```python
from build123d import *

# Parameters (mm, degrees)
F0_W     = 200
F0_H     = 200
F2_DEPTH = 0.5
F1_R     = 10
F3_DEPTH = 10


# Not quite as in the source:
# - a fillet or chamfer that OpenCascade refuses, or shapes differently, is made with other operations: its cross-section is extruded or revolved along the edge and cut away or added


with BuildPart() as f2:
    # F0 (on Top) → F2 (new body)
    with BuildSketch(Plane.XY):
        Rectangle(F0_W, F0_H)
    extrude(amount=F2_DEPTH)

    # F1 (on face) → F3 (join)
    with BuildSketch(Plane.XY):
        with Locations((-55, -20)):
            Circle(F1_R)
        with Locations((-15, 20)):
            Circle(F1_R)
        with Locations((25, -60)):
            Circle(F1_R)
        with Locations((25, 20)):
            Circle(F1_R)
        with Locations((65, -20)):
            Circle(F1_R)
        with Locations((65, 20)):
            Circle(F1_R)
    extrude(amount=F3_DEPTH)

    # F4: fillet of radius 10 on 6 edges, made by hand

    # F4_s1 → F4_t2 (revolve, cut)
    with BuildSketch(Plane.XZ.offset(20)):
        with BuildLine():
            ThreePointArc((-45, 0.5), (-48.0954678017, 7.2456883731), (-54.9874921777, 10))
            Line((-54.9874921777, 10), (-45, 10))
            Line((-45, 10), (-45, 0.5))
        make_face()
    revolve(axis=Axis((-55, -20, 10), (0, 0, 1)), mode=Mode.SUBTRACT)

    # F4_s3 → F4_t4 (revolve, cut)
    with BuildSketch(Plane.XZ.offset(-20)):
        with BuildLine():
            ThreePointArc((-5, 0.5), (-8.0954678017, 7.2456883731), (-14.9874921777, 10))
            Line((-14.9874921777, 10), (-5, 10))
            Line((-5, 10), (-5, 0.5))
        make_face()
    revolve(axis=Axis((-15, 20, 10), (0, 0, 1)), mode=Mode.SUBTRACT)

    # F4_s5 → F4_t6 (revolve, cut)
    with BuildSketch(Plane.XZ.offset(-20)):
        with BuildLine():
            ThreePointArc((35, 0.5), (31.9045321983, 7.2456883731), (25.0125078223, 10))
            Line((25.0125078223, 10), (35, 10))
            Line((35, 10), (35, 0.5))
        make_face()
    revolve(axis=Axis((25, 20, 10), (0, 0, 1)), mode=Mode.SUBTRACT)

    # F4_s7 → F4_t8 (revolve, cut)
    with BuildSketch(Plane.XZ.offset(-20)):
        with BuildLine():
            ThreePointArc((75, 0.5), (71.9045321983, 7.2456883731), (65.0125078223, 10))
            Line((65.0125078223, 10), (75, 10))
            Line((75, 10), (75, 0.5))
        make_face()
    revolve(axis=Axis((65, 20, 10), (0, 0, 1)), mode=Mode.SUBTRACT)

    # F4_s9 → F4_t10 (revolve, cut)
    with BuildSketch(Plane.XZ.offset(20)):
        with BuildLine():
            ThreePointArc((75, 0.5), (71.9045321983, 7.2456883731), (65.0125078223, 10))
            Line((65.0125078223, 10), (75, 10))
            Line((75, 10), (75, 0.5))
        make_face()
    revolve(axis=Axis((65, -20, 10), (0, 0, 1)), mode=Mode.SUBTRACT)

    # F4_s11 → F4_t12 (revolve, cut)
    with BuildSketch(Plane.XZ.offset(60)):
        with BuildLine():
            ThreePointArc((35, 0.5), (31.9045321983, 7.2456883731), (25.0125078223, 10))
            Line((25.0125078223, 10), (35, 10))
            Line((35, 10), (35, 0.5))
        make_face()
    revolve(axis=Axis((25, -60, 10), (0, 0, 1)), mode=Mode.SUBTRACT)


solid = f2.part
```
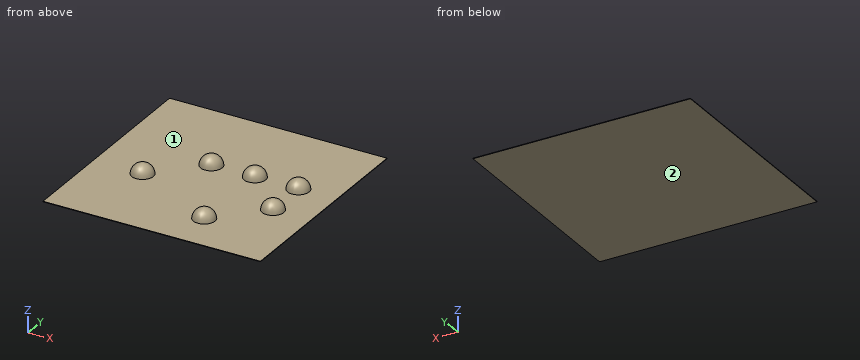
Here's how the part is built. I have some questions about the finished solid (model axes, mm). Face numbers are marked on the shaded views. A direction names the side the tool comes from. Round coordinates to 2 decimals unless told otherwise and drop trailing zeros. Loops run counter-clockwise (first coordinate to the right, second up) from the corner with the lowest first, then second, coordinate; pieces in that order, holes last.
1. Suppose I cut it at B-B, the plane z = 6.5. Give the number of separate pieces and of enclosed holes in the cut face, and give its area (3 significant figures).
Answers:
separate pieces: 6
enclosed holes: 0
area: 1,090 mm2
2. For the marked faces 1 and 2, which set-ups out of +Z, -Z, +X, -X, +Y, -Y let a thin tool reach every point of the face, with its end or its side?
Answers:
face 1: +Z
face 2: -Z, +X, -X, +Y, -Y
3. Suppose I cut it at A-A, the plane y = -1.5. Please give me the cut outline in (x, z), and give its area (3 significant figures).
Answers:
outline: (-100, 0) - (100, 0) - (100, 0.5) - (-100, 0.5) - close
area: 100 mm2
4. If I drill on probe 1 along Z at (x, y) = (68, -1); probe 2 along X at (y, z) = (-17.5, 4.75); probe 3 along Y at (x, z) = (-24, 2), over which ranges is the centre line in solid material (lowest first)?
Answers:
probe 1: z = 0 to 0.5
probe 2: x = -63.45 to -46.55, 56.55 to 73.45
probe 3: y = 16.1 to 23.9
5. Will these pins go through, and if not, where does the flat tip stop? pin 1 (1 mm diameter, centred on y = -66.5, z = 8.5, fed in from +X); pin 2 (5 mm diameter, centred on y = -51, z = 6, fed in from +X); pin 3 (1.5 mm diameter, centred on x = 10.5, y = 73, fed in from +Z).
Answers:
pin 1: passes through
pin 2: stops at x = 30.57
pin 3: stops at z = 0.5
